Autodesk Inventor part; units mm, degrees
ref_plane "YZ Plane" through (0, 0, 0) normal (1, 0, 0) x (0, 1, 0)
ref_plane "XZ Plane" through (0, 0, 0) normal (0, 1, 0) x (-1, 0, 0)
ref_plane "XY Plane" through (0, 0, 0) normal (0, 0, 1) x (1, 0, 0)
sketch "Esquisse1" plane through (0, 0, 0) normal (0, 0, 1) x (1, 0, 0)
  line L0 (-8, -55) -> (8, -55)
  line L1 (10, -53) -> (10, 53)
  line L2 (8, 55) -> (-8, 55)
  line L3 (-10, 53) -> (-10, -53)
  line L4 (-10, -55) -> (10, 55) construction
  line L5 (10, -55) -> (-10, 55) construction
  arc A0 (-8, 55) -> (-10, 53) centre (-8, 53) ccw
  arc A1 (-10, -53) -> (-8, -55) centre (-8, -53) ccw
  arc A2 (8, -55) -> (10, -53) centre (8, -53) ccw
  arc A3 (10, 53) -> (8, 55) centre (8, 53) ccw
  circle A4 centre (0, 45) radius 4.25
  circle A5 centre (0, 25) radius 4.25
  point P0 (0, 0)
  dimension "d0" = 20
  dimension "d1" = 110
  dimension "d2" = 2
  dimension "d3" = 8.5
  dimension "d4" = 8.5
  dimension "d5" = 80
  dimension "d6" = 20
extrude "Extrusion1" add sketch "Esquisse1" against normal blind 5
sketch "Esquisse2" plane through (0, 0, 0) normal (0, 0, 1) x (1, 0, 0)
  circle A0 centre (0, -35) radius 9
  line L0 (-8, -55) -> (8, -55)
  point P0 (0, 0)
  dimension "d9" = 18
  dimension "d10" = 20
extrude "Extrusion2" add sketch "Esquisse2" along normal blind 5
sketch "Esquisse3" plane through (0, -35, 5) normal (0, 0, 1) x (1, 0, 0)
  line L0 (-8, 10) -> (8, 10)
  line L1 (10, 8) -> (10, -8)
  line L2 (8, -10) -> (-8, -10)
  line L3 (-10, -8) -> (-10, 8)
  line L4 (-10, 10) -> (10, -10) construction
  line L5 (10, 10) -> (-10, -10) construction
  arc A0 (-8, 10) -> (-10, 8) centre (-8, 8) ccw
  arc A1 (-10, -8) -> (-8, -10) centre (-8, -8) ccw
  arc A2 (8, -10) -> (10, -8) centre (8, -8) ccw
  arc A3 (10, 8) -> (8, 10) centre (8, 8) ccw
  point P0 (0, 35)
  point P1 (0, 0)
  dimension "d13" = 20
  dimension "d14" = 20
  dimension "d17" = 2
extrude "Extrusion3" add sketch "Esquisse3" along normal blind 35
sketch "Esquisse4" plane through (0, -35, 40) normal (0, 0, 1) x (1, 0, 0)
  arc A0 (3.9626, -15.4418) -> (-3.9626, -15.4418) centre (0, 1.6036) ccw
  arc A1 (3.9626, -15.4418) -> (-3.9626, -15.4418) centre (0, -14.8964) ccw
  point P0 (0, 35)
  dimension "d18" = 35
  dimension "d19" = 8
  dimension "d20" = 16.5
extrude "Extrusion4" add sketch "Esquisse4" along normal blind 6
sketch "Esquisse5" plane through (0, -35, 46) normal (0, 0, 1) x (1, 0, 0)
  arc A0 (3.9626, -15.4418) -> (-3.9626, -15.4418) centre (0, 1.6036) ccw
  point P0 (0, 35)
hole "Perçage1" at (0, -33.3964, 46) direction (0, 0, -1) diameter 6.4008 depth 10 counterbore diameter 12.6 counterbore depth 0
properties part number "SupportTendeurV2"
Here's how the part is built. I have some questions about the finished solid (model axes, mm). A direction names the side the tool comes from. Give positions to 0.01 mm unless a question says otherwise; leave off trailing zeros. Write each loop counter-clockwise with the first axis right and the second up, starting at its lowest first coordinate (ties: lowest second). Pieces come first, ordered by that corner, then holes. Notation, with made-up numbers: M -6,24 L 6,24 A16 cw 6,37 Z; hole C 83.25,-4.5 d7. An arc over 180 degrees is marked long. Put each result on its own line as item: value. Start each with the question number.
Item 1: Thinking about a two-plate mould opening in Y: for faces 6 (the flat face through (0, -55, -2)), 7 (the cylindrical face through (-0.92, 40.85, -2.46)), 8 (the flat face through (0, 55, -2)), which applies, +Y half, -Y half, draft (parallel to the pull), parting line (faces both ways), or undercut?
Item 2: Will these pins go through, and if not, where does the flat tip stop? pin 1 (6 mm diameter, centred on x = 0, z = 28, fed in from +Y); pin 2 (8 mm diameter, centred on y = -37, z = 30.5, fed in from -X); pin 3 (8 mm diameter, centred on x = -3, z = 26.5, fed in from -Y).
Item 3: If we section it at C-C, the plane z = 21: Write out the boundary of the cut face in (x, y), then the cut area to 3 significant figures.
Item 4: On a 3-axis mill with a long thin cutter (end or side, diameter ignored), from which of +Z, -Z, +X, -X, +Y, -Y can I reach the whole of each face in a straight line? I mean faces 1 (the flat face through (0, -25, 22)), 2 (the flat face through (0, -33, 36)), 3 (the cylindrical face through (-1.172, -43.923, 2.465)), 4 (the cylindrical face through (9.43, -44.4, 22.26)), 5 (the flat face through (10, -1, -2)). Say none if no direction works.
Item 5: If we section it at B-B, the plane x = 0: Write out the boundary of the cut face in (y, z), then the cut area to 3 significant figures.
Item 6: I need wall thicknesses on L1, parallel to Y at x = 0, z = -3.35; L2, parallel to Y at x = 0, z = 44; L3, parallel to Y at x = 1, z = -1. Which ranges of each line are inside material? Lowest first, please. Write a range as from..to.
Item 7: If we section it at D-D, the plane y = -18.5: Write out the boundary of the cut face in (x, z), then the cut area to 3 significant figures.
Item 8: If we section it at A-A, the plane y = 45: Write out the boundary of the cut face in (x, z).
Values:
1. face 6: -Y half
1. face 7: undercut
1. face 8: +Y half
2. pin 1: y = -25
2. pin 2: x = -10
2. pin 3: y = -45
3. outline: M -10,-43 A2 ccw -8,-45 L 8,-45 A2 ccw 10,-43 L 10,-27 A2 ccw 8,-25 L -8,-25 A2 ccw -10,-27 Z
3. area: 397 mm²
4. face 1: +X, -X, +Y
4. face 2: +Z
4. face 3: none
4. face 4: +X, -Y
4. face 5: -Z, +X, +Y, -Y
5. outline: M -55,-5 L 20.75,-5 L 20.75,0 L -26,0 L -26,5 L -25,5 L -25,40 L -15.9,40 L -15.9,46 L -30.2,46 L -30.2,36 L -36.6,36 L -36.6,46 L -45.9,46 L -45.9,40 L -45,40 L -45,5 L -44,5 L -44,0 L -55,0 Z; M 29.25,-5 L 40.75,-5 L 40.75,0 L 29.25,0 Z; M 49.25,-5 L 55,-5 L 55,0 L 49.25,0 Z
5. area: 1,370 mm²
6. L1: -55..20.75, 29.25..40.75, 49.25..55
6. L2: -45.9..-36.6, -30.2..-15.9
6. L3: -55..20.87, 29.13..40.87, 49.13..55
7. outline: M -10,-5 L 10,-5 L 10,0 L -10,0 Z; M -9.18,40 L 9.18,40 L 9.18,46 L -9.18,46 Z
7. area: 210 mm²
8. outline: M -10,-5 L -4.25,-5 L -4.25,0 L -10,0 Z; M 4.25,-5 L 10,-5 L 10,0 L 4.25,0 Z
